For this review, take the finished solid that the model builds, in its own axes (mm). A direction names the side the tool comes from. Round coordinates to 2 decimals unless told otherwise and drop trailing zeros. Order: outer loops, then holes, each group sorted by start corner. A loop starts at its lowest first (then second) coordinate and runs counter-clockwise, first axis right, second up. Notation, with made-up numbers: M 9.25,-39 L 38.25,-39 A21 cw 38.25,-25 Z; hole C 4,9.25 d6. An arc over 180 degrees is marked long. Answer in a Markdown table with one row per item. Add a question column.
```python
from build123d import *

# Parameters (mm, degrees)
BASE_DEPTH                = 25.4
BOSS_EXTRUDE1_DEPTH       = 6.35
BOSS_EXTRUDE2_DEPTH       = 6.35
SKETCH7_W                 = 45.72
SKETCH7_H                 = 1.524
BOSS_EXTRUDE3_DEPTH       = 8.89
SKETCH3_W                 = 25.4
SKETCH3_H                 = 5.08
FRONT_SCREW_SUPPORT_DEPTH = 25.4
SKETCH4_R                 = 2.54
CUT_EXTRUDE1_DEPTH        = 5.08
FILLET3_R                 = 10
FILLET4_R                 = 5.08


with BuildPart() as part:
    # Sketch1 → Base (new body)
    with BuildSketch(Plane(origin=(0, 0, 0), x_dir=(0, 0, -1), z_dir=(1, 0, 0))):
        Polygon((0, 0), (0, 5.08), (22.86, 5.08), (22.86, 52.07), (29.21, 52.07), (29.21, 5.08), (72.39, 5.08), (72.39, 52.07), (78.74, 52.07), (78.74, 5.08), (101.6, 5.08), (101.6, 0), align=None)
    extrude(amount=BASE_DEPTH)

    # Sketch5 → Boss-Extrude1 (add)
    with BuildSketch(Plane(origin=(0, 0, -78.74), x_dir=(-1, 0, 0), z_dir=(0, 0, -1))):
        Polygon((-35.56, 52.07), (-35.56, 50.208216501), (-25.4, 38.1), (-25.4, 52.07), (0, 52.07), (0, 38.1), (10.16, 50.208216501), (10.16, 52.07), (10.16, 54.61), (-35.56, 54.61), align=None)
    extrude(amount=-BOSS_EXTRUDE1_DEPTH)

    # Sketch6 → Boss-Extrude2 (add)
    with BuildSketch(Plane.XY.offset(-22.86)):
        Polygon((0, 52.07), (0, 38.1), (-10.16, 50.208216501), (-10.16, 54.61), (35.56, 54.61), (35.56, 50.208216501), (25.4, 38.1), (25.4, 52.07), align=None)
    extrude(amount=-BOSS_EXTRUDE2_DEPTH)

    # Sketch7 → Boss-Extrude3 (add)
    with BuildSketch(Plane.XY.offset(-72.39)):
        with Locations((12.7, 53.848)):
            Rectangle(SKETCH7_W, SKETCH7_H)
    boss_extrude3 = extrude(amount=BOSS_EXTRUDE3_DEPTH)

    # Mirror19: Boss-Extrude3 across plane
    add(boss_extrude3.mirror(Plane.XY.offset(-50.8)))

    # Sketch3 → Front Screw Support (add)
    with BuildSketch(Plane(origin=(25.4, 0, 0), x_dir=(0, 0, -1), z_dir=(1, 0, 0))):
        with Locations((50.8, 2.54)):
            Rectangle(SKETCH3_W, SKETCH3_H)
    front_screw_support = extrude(amount=FRONT_SCREW_SUPPORT_DEPTH)

    # Mirror3: Front Screw Support across plane
    add(front_screw_support.mirror(Plane(origin=(12.7, 0, 0), x_dir=(0, 0, 1), z_dir=(1, 0, 0))))

    # Sketch4 → Cut-Extrude1 (cut)
    with BuildSketch(Plane(origin=(0, 5.08, 0), x_dir=(1, 0, 0), z_dir=(0, 1, 0))):
        with Locations((-17.78, 50.8)):
            Circle(SKETCH4_R)
        with Locations((43.18, 50.8)):
            Circle(SKETCH4_R)
        with Locations((12.7, 93.98)):
            Circle(SKETCH4_R)
        with Locations((12.7, 7.62)):
            Circle(SKETCH4_R)
    extrude(amount=-CUT_EXTRUDE1_DEPTH, mode=Mode.SUBTRACT)

    # Fillet3
    fillet3_edges = [part.edges().sort_by_distance(p)[0] for p in [
        (35.56, 52.40910825, -78.74),
        (-10.16, 52.40910825, -78.74),
        (-10.16, 52.40910825, -22.86),
        (35.56, 52.40910825, -22.86),
    ]]
    fillet(fillet3_edges, radius=FILLET3_R)

    # Fillet4
    fillet4_edges = [part.edges().sort_by_distance(p)[0] for p in [
        (25.4, 2.54, -63.5),
        (25.4, 2.54, -38.1),
        (0, 2.54, -63.5),
        (0, 2.54, -38.1),
        (12.7, 5.08, -22.86),
        (12.7, 5.08, -78.74),
    ]]
    fillet(fillet4_edges, radius=FILLET4_R)


solid = part.part
```
1. Consider section B-B on y = 14. Write out the cut boundary in (x, z), plus the area to 3 significant figures.
2. The part is to be moulded in two halves that separate along Z. For faces 4 (the flat face through (13, 29, -72.39)), 5 (the flat face through (13, 33, -78.74)), 6 (the cylindrical face through (26.849, 2.576, -36.572)), say which applies: pulls with the +Z half, pulls with the -Z half, needs draft (parallel to the pull), parting line crosses it, or undercut.
3. Consider section D-D on z = -50.8. Write out the cut boundary in (x, y).
4. For faces 1 (the flat face through (12, 53.086, -34)), 2 (the flat face through (-15, 3, -63.5)), 3 (the flat face through (13, 33, -22.86)), list the 3-axis set-ups (+Z, -Z, +X, -X, +Y, -Y) from which the entire face can be reached by the end or side of a thin tool; tool diameter is ignored.
5. To check wall thickness, follow probe 1 along X at (y, z) = (2.9, -50.8); probe 2 along Z at (x, y) = (12.7, 3.6); probe 3 along Z at (x, y) = (43.18, 1.8). State the ranges of each line that lie inside material, in increasing order. Write a range as [from, to].
6. Clearance check with flat-ended pins moving along their axes: pin 1 Ø1.2 at (y, z) = (54, -66.5) entering from -X; pin 2 Ø1.5 at (x, y) = (3, 48) entering from +Z; pin 3 Ø3 at (x, z) = (43.18, -50.8) entering from +Y; pin 4 Ø10 at (x, y) = (29.5, 10.5) entering from +Z. State where each tip first meets the part, or that it passes through.
7. Consider section A-A on z = -7.62. Write out the cut boundary in (x, y).
8. Consider section C-C on x = 12.7. Write out the cut boundary in (y, z).
Solved:
| question | item | result |
|---|---|---|
| 1 | outline | M 0,-78.74 L 25.4,-78.74 L 25.4,-72.39 L 0,-72.39 Z; M 0,-29.21 L 25.4,-29.21 L 25.4,-22.86 L 0,-22.86 Z |
| 1 | area | 323 mm^2 |
| 2 | face 4 | undercut |
| 2 | face 5 | pulls with the -Z half |
| 2 | face 6 | pulls with the +Z half |
| 3 | outline | M -25.4,0 L -20.32,0 L -20.32,5.08 L -25.4,5.08 Z; M -15.24,0 L 40.64,0 L 40.64,5.08 L -15.24,5.08 Z; M 45.72,0 L 50.8,0 L 50.8,5.08 L 45.72,5.08 Z |
| 4 | face 1 | +X, -X |
| 4 | face 2 | -Z, -X, -Y |
| 4 | face 3 | +Z, +X, -X, +Y |
| 5 | probe 1 | x = [-25.4, -20.32], [-15.24, 40.64], [45.72, 50.8] |
| 5 | probe 2 | z = [-101.6, -96.52], [-91.44, -10.16], [-5.08, 0] |
| 5 | probe 3 | z = [-63.5, -53.34], [-48.26, -38.1] |
| 6 | pin 1 | stops at x = -10.16 |
| 6 | pin 2 | stops at z = -22.86 |
| 6 | pin 3 | passes through |
| 6 | pin 4 | stops at z = -22.19 |
| 7 | outline | M 0,0 L 10.16,0 L 10.16,5.08 L 0,5.08 Z; M 15.24,0 L 25.4,0 L 25.4,5.08 L 15.24,5.08 Z |
| 8 | outline | M 0,-101.6 L 5.08,-101.6 L 5.08,-96.52 L 0,-96.52 Z; M 0,-91.44 L 5.08,-91.44 L 5.08,-83.82 A5.08 cw 10.16,-78.74 L 54.61,-78.74 L 54.61,-63.5 L 53.09,-63.5 L 53.09,-72.39 L 5.08,-72.39 L 5.08,-29.21 L 53.09,-29.21 L 53.09,-38.1 L 54.61,-38.1 L 54.61,-22.86 L 10.16,-22.86 A5.08 cw 5.08,-17.78 L 5.08,-10.16 L 0,-10.16 Z; M 0,-5.08 L 5.08,-5.08 L 5.08,0 L 0,0 Z |
